The model under review builds one solid part; all positions refer to its coordinate system, in mm. Face numbers are marked on the shaded views. Round coordinates to 2 decimals unless told otherwise and drop trailing zeros. Order: outer loops, then holes, each group sorted by start corner. A loop starts at its lowest first (then second) coordinate and runs counter-clockwise, first axis right, second up.
1) Consider section C-C (x = 7.5). Give the boundary of the cut face in (y, z), then the cut area to 3 significant figures.
2) Mouldability with a two-part tool opening along Y and no side actions: class the marked faces 1, 2 and 3 as pulls with the +Y half, pulls with the -Y half, needs draft (parallel to the pull), parting line crosses it, or undercut.
3) Consider section D-D (y = 6.75). Give the boundary of the cut face in (x, z).
4) To check wall thickness, follow L1, parallel to Z at x = 9, y = -5; L2, parallel to Y at x = 0, z = 17.5; L3, parallel to X at y = 3.25, z = 19.25. State the ranges of each line that lie inside material, in increasing order.
5) Consider section B-B (y = 2.25). Give the boundary of the cut face in (x, z).
6) Consider section A-A (x = 0). Give the boundary of the cut face in (y, z).
7) Clearance check with flat-ended pins moving along their axes: P1, Ø8, axis at y = -2.5, z = 9, coming from the -X side; P2, Ø1.5, axis at x = 2.5, z = 20.5, coming from the -Y side; P3, Ø8, axis at x = 6.5, z = 16, coming from the +Y side; P4, Ø3, axis at y = 7, z = 15, coming from the -X side. State where each tip first meets the part, or that it passes through.
from build123d import *

# Parameters (mm, degrees)
SKETCH1_R           = 10.5
BOSS_EXTRUDE1_DEPTH = 30
SKETCH2_R           = 6
CUT_EXTRUDE1_DEPTH  = 30
CUT_EXTRUDE2_START  = -3
SKETCH3_R           = 10.5
SKETCH3_R_2         = 10
CUT_EXTRUDE2_DEPTH  = 1
CUT_EXTRUDE3_START  = -4
SKETCH4_R           = 10.5
SKETCH4_R_2         = 10
CUT_EXTRUDE3_DEPTH  = 1


with BuildPart() as part:
    # Sketch1 → Boss-Extrude1 (new body)
    with BuildSketch(Plane.XY):
        Circle(SKETCH1_R)
    extrude(amount=BOSS_EXTRUDE1_DEPTH)

    # Sketch2 → Cut-Extrude1 (cut)
    with BuildSketch(Plane(origin=(0, 0, 0), x_dir=(-1, 0, 0), z_dir=(0, 0, -1))):
        with Locations((0, 0.188162924)):
            Circle(SKETCH2_R)
    extrude(amount=-CUT_EXTRUDE1_DEPTH, mode=Mode.SUBTRACT)

    # Sketch3 → Cut-Extrude2 (cut)
    with BuildSketch(Plane(origin=(0, 0, 0), x_dir=(-1, 0, 0), z_dir=(0, 0, -1)).offset(CUT_EXTRUDE2_START)):
        Circle(SKETCH3_R)
        Circle(SKETCH3_R_2, mode=Mode.SUBTRACT)
    extrude(amount=-CUT_EXTRUDE2_DEPTH, mode=Mode.SUBTRACT)

    # Sketch4 → Cut-Extrude3 (cut)
    with BuildSketch(Plane.XY.offset(30).offset(CUT_EXTRUDE3_START)):
        with Locations(Location((0, 0, 0), (0, 0, 180))):
            Circle(SKETCH4_R)
        with Locations(Location((0, 0, 0), (0, 0, 180))):
            Circle(SKETCH4_R_2, mode=Mode.SUBTRACT)
    extrude(amount=CUT_EXTRUDE3_DEPTH, mode=Mode.SUBTRACT)


solid = part.part
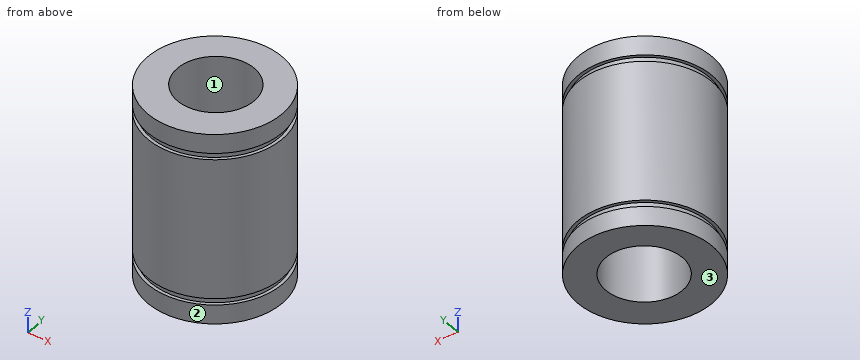
Answer below:
1. outline: (-7.35, 0) - (7.35, 0) - (7.35, 3) - (6.61, 3) - (6.61, 4) - (7.35, 4) - (7.35, 26) - (6.61, 26) - (6.61, 27) - (7.35, 27) - (7.35, 30) - (-7.35, 30) - (-7.35, 27) - (-6.61, 27) - (-6.61, 26) - (-7.35, 26) - (-7.35, 4) - (-6.61, 4) - (-6.61, 3) - (-7.35, 3) - close
1. area: 438 mm2
2. face 1: undercut
2. face 2: parting line crosses it
2. face 3: needs draft
3. outline: (-8.04, 0) - (8.04, 0) - (8.04, 3) - (7.38, 3) - (7.38, 4) - (8.04, 4) - (8.04, 26) - (7.38, 26) - (7.38, 27) - (8.04, 27) - (8.04, 30) - (-8.04, 30) - (-8.04, 27) - (-7.38, 27) - (-7.38, 26) - (-8.04, 26) - (-8.04, 4) - (-7.38, 4) - (-7.38, 3) - (-8.04, 3) - close
4. L1: z = 0 to 3, 4 to 26, 27 to 30
4. L2: y = -10.5 to -5.81, 6.19 to 10.5
4. L3: x = -9.98 to -5.16, 5.16 to 9.98
5. outline: (-10.26, 0) - (-5.63, 0) - (-5.63, 30) - (-10.26, 30) - (-10.26, 27) - (-9.74, 27) - (-9.74, 26) - (-10.26, 26) - (-10.26, 4) - (-9.74, 4) - (-9.74, 3) - (-10.26, 3) - close; (5.63, 0) - (10.26, 0) - (10.26, 3) - (9.74, 3) - (9.74, 4) - (10.26, 4) - (10.26, 26) - (9.74, 26) - (9.74, 27) - (10.26, 27) - (10.26, 30) - (5.63, 30) - close
6. outline: (-10.5, 0) - (-5.81, 0) - (-5.81, 30) - (-10.5, 30) - (-10.5, 27) - (-10, 27) - (-10, 26) - (-10.5, 26) - (-10.5, 4) - (-10, 4) - (-10, 3) - (-10.5, 3) - close; (6.19, 0) - (10.5, 0) - (10.5, 3) - (10, 3) - (10, 4) - (10.5, 4) - (10.5, 26) - (10, 26) - (10, 27) - (10.5, 27) - (10.5, 30) - (6.19, 30) - close
7. P1: stops at x = -10.5
7. P2: stops at y = -10.35
7. P3: stops at y = 10.2
7. P4: stops at x = -8.94
